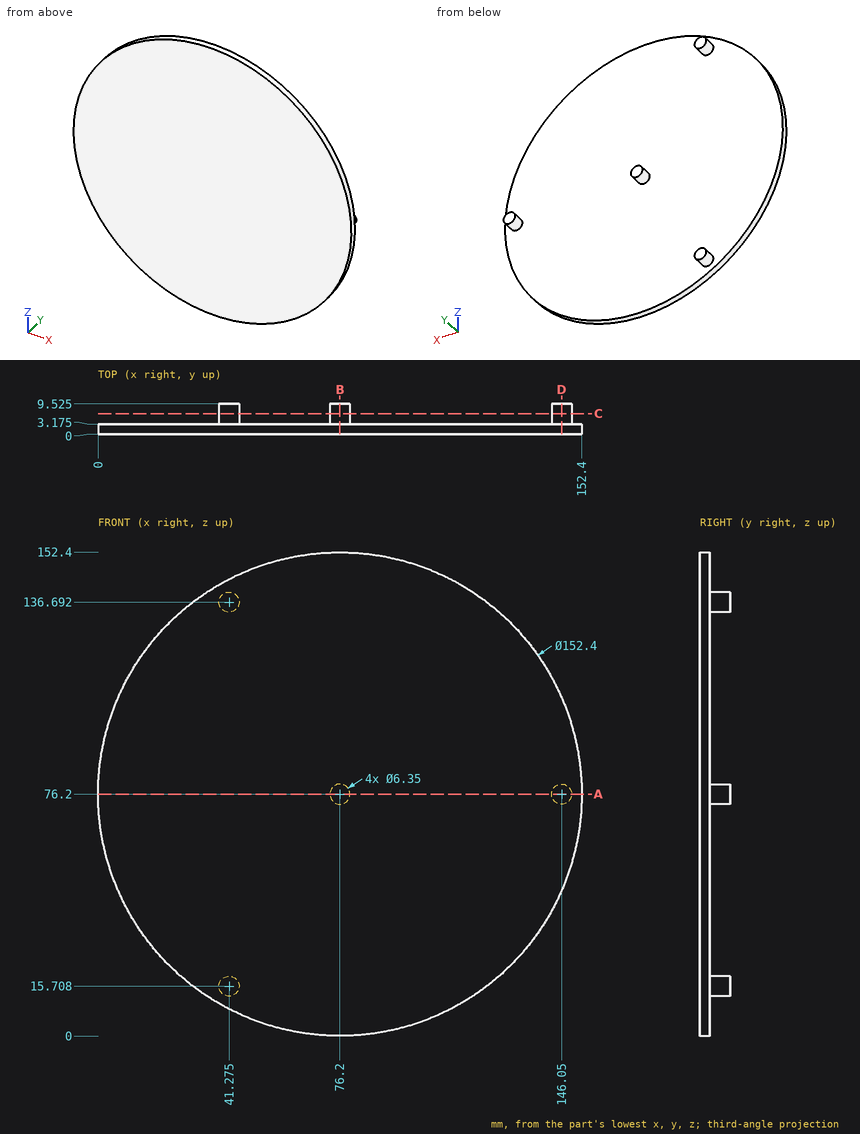
Input: dimensioned drawing with shaded views. Units: mm. Origin: part minimum x, y, z. Give positions to 0.01 mm unless a question says otherwise; leave off trailing zeros. Order: outer loops, then holes, each group sorted by start corner. A loop starts at its lowest first (then second) coordinate and runs counter-clockwise, first axis right, second up. Notation, with made-up numbers: (30.5, -6) -> (75.5, -6) arc R23 ccw to (75.5, 29) -> close; hole circle Ø3 at (54.5, -2). An arc over 180 degrees is marked (long way). Use one line per item in the form item = value.
1) Section A-A, the plane z = 76.2. Return loops of the section in (x, y) (3 decimals).
Response values:
outline = (0, 0) -> (152.4, 0) -> (152.4, 3.175) -> (149.225, 3.175) -> (149.225, 9.525) -> (142.875, 9.525) -> (142.875, 3.175) -> (79.375, 3.175) -> (79.375, 9.525) -> (73.025, 9.525) -> (73.025, 3.175) -> (0, 3.175) -> close
2) Section D-D, the plane x = 146.05. Return loops of the section in (y, z) (1 decimal).
Response values:
outline = (0, 45.7) -> (3.2, 45.7) -> (3.2, 73) -> (9.5, 73) -> (9.5, 79.4) -> (3.2, 79.4) -> (3.2, 106.7) -> (0, 106.7) -> close
3) First-contact query: pin 1 Ø2 at (x, y) = (112.5, 3) entering from +Z; pin 2 Ø3 at (y, z) = (3, 55) entering from -X; pin 3 Ø1.5 at (y, z) = (2, 41.5) entering from -X; pin 4 Ø3 at (x, z) = (113.5, 108.5) entering from -Y. Flat tips, straight axial feed; report the tip coordinate or a pass-through.
Response values:
pin_1 = 143.73
pin_2 = 2.59
pin_3 = 7.98
pin_4 = 0
4) Line query: probe 1 along Y at (x, z) = (99, 39) (3 decimals); probe 2 along Z at (x, y) = (75, 1.75); probe 3 along X at (y, z) = (8, 134.5). Output: solid intervals per line, ascending.
Response values:
probe_1 = 0 to 3.175
probe_2 = 0.01 to 152.39
probe_3 = 38.98 to 43.57
5) Section C-C, the plane y = 6.5. Count the separate pieces of the cut face and the enclosed holes in it, and give its area (3 significant figures).
Response values:
separate_pieces = 4
enclosed_holes = 0
area = 127 mm^2
6) Section B-B, the plane x = 76.2. Return loops of the section in (y, z) (3 decimals), and give its area (3 significant figures).
Response values:
outline = (0, 0) -> (3.175, 0) -> (3.175, 73.025) -> (9.525, 73.025) -> (9.525, 79.375) -> (3.175, 79.375) -> (3.175, 152.4) -> (0, 152.4) -> close
area = 524 mm^2
